```python
from build123d import *

# Parameters (mm, degrees)
SKETCH1_R           = 3.4
BOSS_EXTRUDE1_DEPTH = 300


with BuildPart() as part:
    # Sketch1 → Boss-Extrude1 (new body)
    with BuildSketch(Plane(origin=(0, 100, 0), x_dir=(1, 0, 0), z_dir=(0, 1, 0))):
        with BuildLine():
            Line((27.5, 0), (20.200000224, 0))
            Line((20.200000224, 0), (20.200000224, -1.1))
            Line((20.200000224, -1.1), (19.1, -1.1))
            Line((19.1, -1.1), (19.1, -2.2))
            Line((19.1, -2.2), (23.249999989, -2.2))
            Line((23.249999989, -2.2), (23.249999989, -5.335786427))
            Line((23.249999989, -5.335786427), (19.385786417, -9.2))
            Line((19.385786417, -9.2), (10.614213562, -9.2))
            Line((10.614213562, -9.2), (6.75, -5.335786438))
            Line((6.75, -5.335786438), (6.75, -2.2))
            Line((6.75, -2.2), (10.9, -2.2))
            Line((10.9, -2.2), (10.9, -1.1))
            Line((10.9, -1.1), (9.799999776, -1.1))
            Line((9.799999776, -1.1), (9.799999776, 0))
            Line((9.799999776, 0), (2.5, 0))
            ThreePointArc((2.5, 0), (0.732233047, -0.732233047), (0, -2.5))
            Line((0, -2.5), (0, -9.799999776))
            Line((0, -9.799999776), (1.1, -9.799999776))
            Line((1.1, -9.799999776), (1.1, -10.9))
            Line((1.1, -10.9), (2.199999979, -10.9))
            Line((2.199999979, -10.9), (2.199999979, -6.750000011))
            Line((2.199999979, -6.750000011), (5.335786427, -6.750000011))
            Line((5.335786427, -6.750000011), (9.199999989, -10.614213573))
            Line((9.199999989, -10.614213573), (9.199999989, -19.385786427))
            Line((9.199999989, -19.385786427), (5.335786417, -23.25))
            Line((5.335786417, -23.25), (2.199999979, -23.25))
            Line((2.199999979, -23.25), (2.199999979, -19.1))
            Line((2.199999979, -19.1), (1.1, -19.1))
            Line((1.1, -19.1), (1.1, -20.200000224))
            Line((1.1, -20.200000224), (0, -20.200000224))
            Line((0, -20.200000224), (0, -27.5))
            ThreePointArc((0, -27.5), (0.732233047, -29.267766953), (2.5, -30))
            Line((2.5, -30), (9.799999776, -30))
            Line((9.799999776, -30), (9.799999776, -28.9))
            Line((9.799999776, -28.9), (10.9, -28.9))
            Line((10.9, -28.9), (10.9, -27.8))
            Line((10.9, -27.8), (6.75, -27.8))
            Line((6.75, -27.8), (6.75, -24.664213562))
            Line((6.75, -24.664213562), (10.614213562, -20.8))
            Line((10.614213562, -20.8), (19.385786417, -20.8))
            Line((19.385786417, -20.8), (23.249999989, -24.664213573))
            Line((23.249999989, -24.664213573), (23.249999989, -27.8))
            Line((23.249999989, -27.8), (19.1, -27.8))
            Line((19.1, -27.8), (19.1, -28.9))
            Line((19.1, -28.9), (20.200000224, -28.9))
            Line((20.200000224, -28.9), (20.200000224, -30))
            Line((20.200000224, -30), (27.5, -30))
            ThreePointArc((27.5, -30), (29.267766953, -29.267766953), (30, -27.5))
            Line((30, -27.5), (30, -20.200000224))
            Line((30, -20.200000224), (28.9, -20.200000224))
            Line((28.9, -20.200000224), (28.9, -19.1))
            Line((28.9, -19.1), (27.799999979, -19.1))
            Line((27.799999979, -19.1), (27.799999979, -23.25))
            Line((27.799999979, -23.25), (24.664213562, -23.25))
            Line((24.664213562, -23.25), (20.799999989, -19.385786427))
            Line((20.799999989, -19.385786427), (20.799999989, -10.614213573))
            Line((20.799999989, -10.614213573), (24.664213552, -6.750000011))
            Line((24.664213552, -6.750000011), (27.799999979, -6.750000011))
            Line((27.799999979, -6.750000011), (27.799999979, -10.9))
            Line((27.799999979, -10.9), (28.9, -10.9))
            Line((28.9, -10.9), (28.9, -9.799999776))
            Line((28.9, -9.799999776), (30, -9.799999776))
            Line((30, -9.799999776), (30, -2.5))
            ThreePointArc((30, -2.5), (29.267766953, -0.732233047), (27.5, 0))
        make_face()
        with Locations((15, -15)):
            Circle(SKETCH1_R, mode=Mode.SUBTRACT)
        with BuildLine():
            Line((28.5, -25.9), (28.5, -27.35))
            ThreePointArc((28.5, -27.35), (28.163172798, -28.163172798), (27.35, -28.5))
            Line((27.35, -28.5), (25.9, -28.5))
            ThreePointArc((25.9, -28.5), (25.086827202, -28.163172798), (24.75, -27.35))
            Line((24.75, -27.35), (24.75, -25.9))
            ThreePointArc((24.75, -25.9), (25.086827202, -25.086827202), (25.9, -24.75))
            Line((25.9, -24.75), (27.35, -24.75))
            ThreePointArc((27.35, -24.75), (28.163172798, -25.086827202), (28.5, -25.9))
        make_face(mode=Mode.SUBTRACT)
        with BuildLine():
            Line((1.5, -27.35), (1.5, -25.9))
            ThreePointArc((1.5, -25.9), (1.836827202, -25.086827202), (2.65, -24.75))
            Line((2.65, -24.75), (4.1, -24.75))
            ThreePointArc((4.1, -24.75), (4.913172798, -25.086827202), (5.25, -25.9))
            Line((5.25, -25.9), (5.25, -27.35))
            ThreePointArc((5.25, -27.35), (4.913172798, -28.163172798), (4.1, -28.5))
            Line((4.1, -28.5), (2.65, -28.5))
            ThreePointArc((2.65, -28.5), (1.836827202, -28.163172798), (1.5, -27.35))
        make_face(mode=Mode.SUBTRACT)
        with BuildLine():
            Line((2.65, -1.5), (4.1, -1.5))
            ThreePointArc((4.1, -1.5), (4.913172798, -1.836827202), (5.25, -2.65))
            Line((5.25, -2.65), (5.25, -4.1))
            ThreePointArc((5.25, -4.1), (4.913172798, -4.913172798), (4.1, -5.25))
            Line((4.1, -5.25), (2.65, -5.25))
            ThreePointArc((2.65, -5.25), (1.836827202, -4.913172798), (1.5, -4.1))
            Line((1.5, -4.1), (1.5, -2.65))
            ThreePointArc((1.5, -2.65), (1.836827202, -1.836827202), (2.65, -1.5))
        make_face(mode=Mode.SUBTRACT)
        with BuildLine():
            Line((28.5, -2.65), (28.5, -4.1))
            ThreePointArc((28.5, -4.1), (28.163172798, -4.913172798), (27.35, -5.25))
            Line((27.35, -5.25), (25.9, -5.25))
            ThreePointArc((25.9, -5.25), (25.086827202, -4.913172798), (24.75, -4.1))
            Line((24.75, -4.1), (24.75, -2.65))
            ThreePointArc((24.75, -2.65), (25.086827202, -1.836827202), (25.9, -1.5))
            Line((25.9, -1.5), (27.35, -1.5))
            ThreePointArc((27.35, -1.5), (28.163172798, -1.836827202), (28.5, -2.65))
        make_face(mode=Mode.SUBTRACT)
    extrude(amount=-BOSS_EXTRUDE1_DEPTH)


solid = part.part
```
Here's how the part is built. I have some questions about the finished solid (model axes, mm). Give positions to 0.01 mm unless a question says otherwise; leave off trailing zeros. Order: outer loops, then holes, each group sorted by start corner. A loop starts at its lowest first (then second) coordinate and runs counter-clockwise, first axis right, second up. Notation, with made-up numbers: (43.5, 63.25) - (91.5, 63.25) arc R27 cw to (91.5, 94.25) - close; hole circle Ø9 at (-32, -18). An arc over 180 degrees is marked (long way). Answer as a JSON object with one key per item and string values. Group by question number.
Item 1: If we section it at C-C on y = -73: Give the number of separate pieces and of enclosed holes in the cut face, and give its area (3 significant figures).
Item 2: If we mould it in two halves opening along X, with no side actions, what happens to faces 1 (the flat face through (15, -48, 20.8)), 2 (the flat face through (0, -48, 24)), 3 (the flat face through (15, -200, 11))? For each: pulls with the +X half, pulls with the -X half, needs draft (parallel to the pull), parting line crosses it, or undercut.
Item 3: For P1, Ø2, axis at y = -44, z = 11, coming from the +X side; P2, Ø1.5, axis at x = 4, z = 22, coming from the -Y side; P3, Ø1, axis at y = -129.5, z = 12.5, coming from the -X side, each with a flat end and sliding along its axis, tell me the tip position at first contact or that it passes through.
Item 4: If we section it at A-A on z = 15: Please give me the cut outline in (x, y).
Item 5: Please list where these lines run through material, in increasing order: probe 1 along X at (y, z) = (49.5, 4.25); probe 2 along X at (y, z) = (-39.5, 15).
Item 6: If we section it at B-B on x = 15: Please give me the cut outline in (y, z), and give its area (3 significant figures).
Result set:
{
 "1": {"separate pieces": "1", "enclosed holes": "5", "area": "322 mm²"},
 "2": {"face 1": "undercut", "face 2": "pulls with the -X half", "face 3": "needs draft"},
 "3": {"P1": "x = 28.9", "P2": "through", "P3": "x = 9.2"},
 "4": {"outline": "(9.2, -200) - (11.6, -200) - (11.6, 100) - (9.2, 100) - close; (18.4, -200) - (20.8, -200) - (20.8, 100) - (18.4, 100) - close"},
 "5": {"probe 1": "0 to 1.51, 5.24 to 6.75, 23.25 to 24.76, 28.49 to 30", "probe 2": "9.2 to 11.6, 18.4 to 20.8"},
 "6": {"outline": "(-200, 9.2) - (100, 9.2) - (100, 11.6) - (-200, 11.6) - close; (-200, 18.4) - (100, 18.4) - (100, 20.8) - (-200, 20.8) - close", "area": "1,440 mm²"}
}
